Autodesk Inventor part; units mm, degrees
ref_plane "YZ Plane" through (0, 0, 0) normal (1, 0, 0) x (0, 1, 0)
ref_plane "XZ Plane" through (0, 0, 0) normal (0, 1, 0) x (-1, 0, 0)
ref_plane "XY Plane" through (0, 0, 0) normal (0, 0, 1) x (1, 0, 0)
sketch "Sketch1" plane through (0, 0, 0) normal (0, 0, 1) x (1, 0, 0)
  circle A0 centre (0, 0) radius 4
  circle A1 centre (0, 0) radius 11
  dimension "d0" = 8
  dimension "d1" = 22
extrude "Extrusion1" add sketch "Sketch1" along normal blind 7
sketch "Sketch2" plane through (0, 0, 7) normal (0, 0, 1) x (1, 0, 0)
  circle A0 centre (0, 0) radius 11
  circle A1 centre (0, 0) radius 12.5
  dimension "d4" = 25
extrude "Extrusion2" add sketch "Sketch2" against normal blind 1.5
sketch "Sketch3" plane through (0, 0, 0) normal (0, 0, -1) x (-1, 0, 0)
  circle A0 centre (0, 0) radius 11
  circle A1 centre (0, 0) radius 5.5937
  circle A2 centre (0, 0) radius 7.0513
extrude "Extrusion3" cut sketch "Sketch3" against normal blind 0.1 contours A2
properties part number "30169-01" material "Steel, Mild"
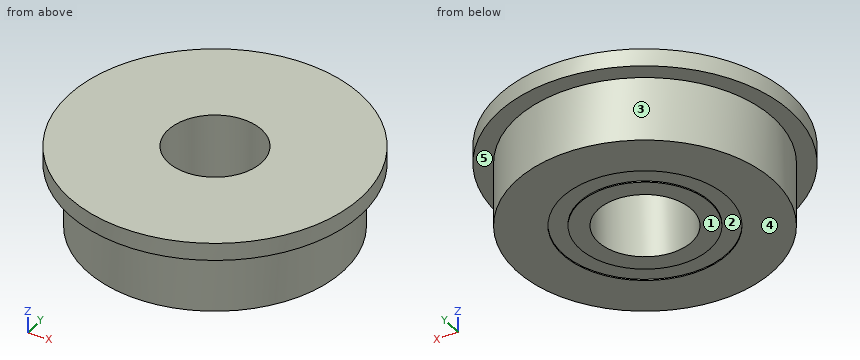
The listing builds one solid part. Answer for the finished solid, in the listing's coordinates (mm). Face numbers are marked on the shaded views. A direction names the side the tool comes from. Round coordinates to 2 decimals unless told otherwise and drop trailing zeros. Order: outer loops, then holes, each group sorted by start corner. A loop starts at its lowest first (then second) coordinate and runs counter-clockwise, first axis right, second up. Notation, with made-up numbers: M 34,84 L 67,84 A15 ccw 67,108 Z; hole C -22,8.25 d2. An arc over 180 degrees is marked long. Answer in a Markdown table with one row per item. Add a question column.
1) Consider line 1 along Y through (x, z) = (0, 3); line 2 along Z through (x, y) = (3.5, -10.5); line 3 along Y through (x, z) = (-1.5, 5). Determine where each line is inside the solid, lowest interval first. Write a range as from..to.
2) Flat-ended cylindrical pins translate along their axes: pin 1 Ø4 at (y, z) = (2.5, 3) entering from -X; pin 2 Ø4 at (y, z) = (6, 6) entering from +X; pin 3 Ø1.5 at (x, z) = (10, 1.5) entering from -Y. Find the tip coordinate at first contact, or state that the pin passes through.
3) Determine the mould class of the marked faces 1, 2 and 3 for opening direction Y: pulls with the +Y half, pulls with the -Y half, needs draft (parallel to the pull), parting line crosses it, or undercut.
4) The part is cut by section D-D on x = -10. Determine the outline of the cut face in (y, z).
5) The part is cut by section C-C on z = 6.25. Determine the outline of the cut face in (x, y), plus the area to 3 significant figures.
6) Which of the six approach directions +Z, -Z, +X, -X, +Y, -Y give full straight-line access (tool end or side, diameter ignored) to the marked faces 4 and 5?
7) The part is cut by section A-A on y = 0. Determine the outline of the cut face in (x, z), plus the area to 3 significant figures.
Findings below:
| question | item | result |
|---|---|---|
| 1 | line 1 | y = -11..-4, 4..11 |
| 1 | line 2 | z = 5.5..7 |
| 1 | line 3 | y = -10.9..-3.71, 3.71..10.9 |
| 2 | pin 1 | stops at x = -10.99 |
| 2 | pin 2 | stops at x = 11.84 |
| 2 | pin 3 | stops at y = -5.95 |
| 3 | face 1 | needs draft |
| 3 | face 2 | undercut |
| 3 | face 3 | parting line crosses it |
| 4 | outline | M -7.5,5.5 L -4.58,5.5 L -4.58,0 L 4.58,0 L 4.58,5.5 L 7.5,5.5 L 7.5,7 L -7.5,7 Z |
| 5 | outline | C 0,0 d25; hole C 0,0 d8 |
| 5 | area | 441 mm² |
| 6 | face 4 | -Z, +X, -X, +Y, -Y |
| 6 | face 5 | -Z |
| 7 | outline | M -12.5,5.5 L -11,5.5 L -11,0 L -7.05,0 L -7.05,0.1 L -5.59,0.1 L -5.59,0 L -4,0 L -4,7 L -12.5,7 Z; M 4,0 L 5.59,0 L 5.59,0.1 L 7.05,0.1 L 7.05,0 L 11,0 L 11,5.5 L 12.5,5.5 L 12.5,7 L 4,7 Z |
| 7 | area | 102 mm² |
